Part model, mm, in its own coordinate system. A direction names the side the tool comes from. Give positions to 0.01 mm unless a question says otherwise; leave off trailing zeros. Loops run counter-clockwise (first coordinate to the right, second up) from the corner with the lowest first, then second, coordinate; pieces in that order, holes last. Notation, with made-up numbers: M 59.5,-19 L 99.5,-19 A32 cw 99.5,18 Z; hole C 6.25,39.25 d1. An arc over 180 degrees is marked long. Answer in a Markdown table with one row per item.
from build123d import *

# Parameters (mm, degrees)
BOSS_EXTRUDE1_DEPTH     = 50.8
SKETCH3_W               = 40
SKETCH3_H               = 45
CUT_EXTRUDE1_DEPTH      = 20
SKETCH4_R               = 2.4892
CUT_EXTRUDE2_DEPTH      = 17.78
SKETCH7_W               = 25.4
SKETCH7_H               = 25.4
CUT_EXTRUDE3_DEPTH      = 19.05
CUT_EXTRUDE4_DEPTH      = 119.867767025
CUT_EXTRUDE4_DEPTH_BACK = 119.867767025
SKETCH10_R              = 2.4892
CUT_EXTRUDE5_DEPTH      = 121.594574863
SKETCH11_R              = 2.54
BOSS_EXTRUDE2_DEPTH     = 5.08


with BuildPart() as part:
    # Sketch1 → Boss-Extrude1 (new body)
    with BuildSketch(Plane.XY):
        Polygon((0, 0), (0, -95.581585113), (-6.35, -95.581585113), (-6.35, -76.531585113), (-59.515515832, -64.891735517), (-35.66310566, 0.642222829), (-6.35, 12.368414887), (-6.35, 31.418414887), (0, 31.418414887), align=None)
    extrude(amount=BOSS_EXTRUDE1_DEPTH)

    # Sketch3 → Cut-Extrude1 (cut)
    with BuildSketch(Plane(origin=(-31.697721226, 11.53702702, 0), x_dir=(0, 0, 1), z_dir=(-0.9396926207859081, 0.34202014332566955, 0))):
        with Locations((25.4, -46.13379027)):
            Rectangle(SKETCH3_W, SKETCH3_H)
    extrude(amount=-CUT_EXTRUDE1_DEPTH, mode=Mode.SUBTRACT)

    # Sketch4 → Cut-Extrude2 (cut)
    with BuildSketch(Plane(origin=(-31.697721226, 11.53702702, 0), x_dir=(0, 0, 1), z_dir=(-0.9396926207859081, 0.34202014332566955, 0))):
        with Locations(Location((25.4, -17.28379027, 0), (0, 0, 270))):
            Circle(SKETCH4_R)
        with Locations(Location((25.4, -74.98379027, 0), (0, 0, 270))):
            Circle(SKETCH4_R)
    extrude(amount=-CUT_EXTRUDE2_DEPTH, mode=Mode.SUBTRACT)

    # Sketch7 → Cut-Extrude3 (cut)
    with BuildSketch(Plane(origin=(-12.90386881, 4.696624154, 0), x_dir=(0, 0, 1), z_dir=(-0.9396926207859082, 0.34202014332566955, 0))):
        with Locations((25.4, -46.13379027)):
            Rectangle(SKETCH7_W, SKETCH7_H)
    extrude(amount=-CUT_EXTRUDE3_DEPTH, mode=Mode.SUBTRACT)

    # Sketch9 → Cut-Extrude4 (cut, two sides: drawn at the far end of the back side and taken through both)
    with BuildSketch(Plane(origin=(0, 0, 38.1), x_dir=(-1, 0, 0), z_dir=(0, 0, -1)).offset(-CUT_EXTRUDE4_DEPTH_BACK)):
        Polygon((6.437754125, -33.236345579), (15.125065765, -57.104538146), (27.059162049, -52.760882326), (18.371850409, -28.892689758), align=None)
    extrude(amount=CUT_EXTRUDE4_DEPTH + CUT_EXTRUDE4_DEPTH_BACK, mode=Mode.SUBTRACT)

    # Sketch10 → Cut-Extrude5 (cut, through all)
    with BuildSketch(Plane.ZY.offset(6.35)):
        with Locations(Location((25.4, 18.718414887, 0), (0, 0, 270))):
            Circle(SKETCH10_R)
        with Locations(Location((12.7, 18.718414887, 0), (0, 0, 270))):
            Circle(SKETCH10_R)
        with Locations(Location((12.7, -82.881585113, 0), (0, 0, 270))):
            Circle(SKETCH10_R)
        with Locations(Location((38.1, -82.881585113, 0), (0, 0, 270))):
            Circle(SKETCH10_R)
        with Locations(Location((38.1, 18.718414887, 0), (0, 0, 270))):
            Circle(SKETCH10_R)
        with Locations(Location((25.4, -82.881585113, 0), (0, 0, 270))):
            Circle(SKETCH10_R)
    extrude(amount=-CUT_EXTRUDE5_DEPTH, mode=Mode.SUBTRACT)

    # Sketch11 → Boss-Extrude2 (add)
    with BuildSketch(Plane(origin=(-12.90386881, 4.696624154, 0), x_dir=(0, 0, 1), z_dir=(-0.9396926207859081, 0.3420201433256697, 0))):
        with Locations(Location((10.48, -28.71379027, 0), (0, 0, 90))):
            Circle(SKETCH11_R)
        with Locations(Location((40.32, -28.71379027, 0), (0, 0, 90))):
            Circle(SKETCH11_R)
        with Locations(Location((40.32, -63.55379027, 0), (0, 0, 90))):
            Circle(SKETCH11_R)
        with Locations(Location((10.48, -63.55379027, 0), (0, 0, 90))):
            Circle(SKETCH11_R)
    extrude(amount=BOSS_EXTRUDE2_DEPTH)


solid = part.part
(1) Saw through at B-B (y = -43). Write the cut outline in (x, z).
Recorded:
| item | result |
|---|---|
| outline | M -51.55,0 L -23.51,0 L -23.51,12.7 L -30.26,12.7 L -30.26,5.4 L -51.55,5.4 Z; M -51.55,45.4 L -30.26,45.4 L -30.26,38.1 L -23.51,38.1 L -23.51,50.8 L -51.55,50.8 Z; M -9.99,0 L 0,0 L 0,50.8 L -9.99,50.8 Z |
(2) Pin check, flat tips, straight feed: pin 1 Ø15 at (y, z) = (-87.5, 36.5) entering from -X; pin 2 Ø21 at (y, z) = (18.5, 19.5) entering from -X; pin 3 Ø3 at (y, z) = (-20, 18.5) entering from -X. Stop position of each tip, or through.
Recorded:
| item | result |
|---|---|
| pin 1 | stops at x = -6.35 |
| pin 2 | stops at x = -17.27 |
| pin 3 | stops at x = -22.44 |
(3) Saw through at C-C (z = 25.4). Give the number of separate pieces and of enclosed holes in the cut face, plus the area to 3 significant figures.
Recorded:
| item | result |
|---|---|
| separate pieces | 3 |
| enclosed holes | 0 |
| area | 2,370 mm^2 |
(4) Pull direction Y, two halves, no side cores. Call faces 1 (the face through (-6.35, -86, 25)), 2 (the face through (-30.516, -14.044, 25.12)), 3 (the face through (-55.707, -54.428, 25.044)), 4 (the face through (-32.561, -70.793, 25.044)): +Y half, -Y half, draft (parallel to the pull), parting line (faces both ways), or undercut.
Recorded:
| item | result |
|---|---|
| face 1 | draft |
| face 2 | undercut |
| face 3 | +Y half |
| face 4 | -Y half |
(5) Saw through at A-A (x = -5). Write the cut outline in (y, z).
Recorded:
| item | result |
|---|---|
| outline | M -95.58,0 L 31.42,0 L 31.42,50.8 L -95.58,50.8 Z; hole C -82.88,12.7 d4.98; hole C -82.88,25.4 d4.98; hole C -82.88,38.1 d4.98; hole C 18.72,12.7 d4.98; hole C 18.72,25.4 d4.98; hole C 18.72,38.1 d4.98 |
(6) Which spindle directions (+Z, -Z, +X, -X, +Y, -Y) get a long thin tool onto all of the face, cutting with end or side? Do faces 5 (the face through (-22.776, -40.994, 44.539)), 6 (the face through (-28.575, -38.359, 38.453)), 7 (the face through (-27.51, -20.58, 10.44)). Say none if no direction does.
Recorded:
| item | result |
|---|---|
| face 5 | +Z, -Z |
| face 6 | none |
| face 7 | -X |
(7) Drill centre lines: line 1 along Y through (x, z) = (-1, 38); line 2 along Y through (x, z) = (-5, 36); line 3 along Z through (x, y) = (-37, -5.5). Where is each one in solid material? Low to high.
Recorded:
| item | result |
|---|---|
| line 1 | y = -95.58 to -85.37, -80.39 to 16.23, 21.21 to 31.42 |
| line 2 | y = -95.58 to -84.22, -81.55 to 17.38, 20.05 to 31.42 |
| line 3 | z = 0 to 22.97, 27.83 to 50.8 |
